Autodesk Fusion 360 part; units mm, degrees
sketch "Skizze1" plane through (0, 0, 0) normal (0, 0, 1) x (1, 0, 0)
  line L0 (-6.5, 4.75) -> (6.5, 4.75)
  line L1 (8.5, 2.75) -> (8.5, -2.75)
  line L2 (6.5, -4.75) -> (-6.5, -4.75)
  line L3 (-8.5, -2.75) -> (-8.5, 2.75)
  line L4 (-8.5, 4.75) -> (8.5, -4.75) construction
  line L5 (8.5, 4.75) -> (-8.5, -4.75) construction
  arc A0 (8.5, 2.75) -> (6.5, 4.75) centre (6.5, 2.75) ccw
  arc A1 (-6.5, 4.75) -> (-8.5, 2.75) centre (-6.5, 2.75) ccw
  arc A2 (-8.5, -2.75) -> (-6.5, -4.75) centre (-6.5, -2.75) ccw
  arc A3 (6.5, -4.75) -> (8.5, -2.75) centre (6.5, -2.75) ccw
  dimension "d464" = 17
  dimension "d465" = 9.5
  dimension "d468" = 2
extrude "Extrusion1" add sketch "Skizze1" along normal blind 2
sketch "Skizze2" plane through (0, 0, 2) normal (0, 0, 1) x (-1, 0, 0)
  arc A0 (8.5, 2.75) -> (6.5, 4.75) centre (6.5, 2.75) ccw
  line L0 (6.5, 4.75) -> (-6.5, 4.75)
  arc A1 (-6.5, 4.75) -> (-8.5, 2.75) centre (-6.5, 2.75) ccw
  line L1 (-8.5, 2.75) -> (-8.5, -2.75)
  arc A2 (-8.5, -2.75) -> (-6.5, -4.75) centre (-6.5, -2.75) ccw
  line L2 (-6.5, -4.75) -> (6.5, -4.75)
  arc A3 (6.5, -4.75) -> (8.5, -2.75) centre (6.5, -2.75) ccw
  line L3 (8.5, -2.75) -> (8.5, 2.75)
  line L4 (3.75, 2.25) -> (-3.75, 2.25)
  line L5 (-3.75, 2.25) -> (-3.75, -2.25)
  line L6 (-3.75, -2.25) -> (3.75, -2.25)
  line L7 (3.75, -2.25) -> (3.75, 2.25)
  line L8 (3.75, 2.25) -> (-3.75, -2.25) construction
  line L9 (-3.75, 2.25) -> (3.75, -2.25) construction
  dimension "d469" = 7.5
  dimension "d470" = 4.5
extrude "Extrusion2" add sketch "Skizze2" along normal blind 10 contours L4 L5 L6 L7
sketch "Skizze3" plane through (0, -2.25, 0) normal (0, -1, 0) x (1, 0, 0)
  line L0 (-3.75, 2) -> (3.75, 2)
  line L1 (3.75, 2) -> (3.75, 12)
  line L2 (3.75, 12) -> (-3.75, 12)
  line L3 (-3.75, 12) -> (-3.75, 2)
  line L4 (-0.875, 12) -> (0.875, 12)
  line L5 (0.875, 12) -> (0.875, 9)
  line L6 (0.875, 9) -> (-0.875, 9)
  line L7 (-0.875, 9) -> (-0.875, 12)
  line L8 (-0.875, 12) -> (0.875, 9) construction
  line L9 (0.875, 12) -> (-0.875, 9) construction
  line L10 (-3.75, 3.25) -> (-2.75, 4.25)
  line L11 (-3.75, 3.25) -> (-1.5, 3.25) construction
  line L12 (-2.75, 4.25) -> (-2.75, 5.75)
  line L13 (-2.75, 5.75) -> (-3.75, 6.75)
  line L14 (-6.5, 2) -> (6.5, 2)
  line L15 (0, 20) -> (0, 2.5)
  line L16 (3.75, 3.25) -> (2.75, 4.25)
  line L17 (2.75, 4.25) -> (2.75, 5.75)
  line L18 (2.75, 5.75) -> (3.75, 6.75)
  point P0 (0, 10.5)
  dimension "d479" = 1.75
  dimension "d480" = 3
  dimension "d483" = 45
  dimension "d484" = 1
  dimension "d485" = 1.5
  dimension "d486" = 2.25
extrude "Extrusion3" cut sketch "Skizze3" against normal up to surface (4.5 mm away) contours L3 L10 L12 L13 | L1 L16 L17 L18 | L2 L4 L6 L7 L15 | L2 L4 L5 L6 L15
sketch "Skizze4" plane through (0, 0, 0) normal (0, 0, -1) x (1, 0, 0)
  arc A0 (-6.5, 4.75) -> (-8.5, 2.75) centre (-6.5, 2.75) ccw
  line L0 (-8.5, 2.75) -> (-8.5, -2.75)
  arc A1 (-8.5, -2.75) -> (-6.5, -4.75) centre (-6.5, -2.75) ccw
  line L1 (-6.5, -4.75) -> (6.5, -4.75)
  arc A2 (6.5, -4.75) -> (8.5, -2.75) centre (6.5, -2.75) ccw
  line L2 (8.5, -2.75) -> (8.5, 2.75)
  arc A3 (8.5, 2.75) -> (6.5, 4.75) centre (6.5, 2.75) ccw
  line L3 (6.5, 4.75) -> (-6.5, 4.75)
  line L4 (-1, 3.5) -> (1, 3.5)
  line L5 (1, 3.5) -> (1, -3.5)
  line L6 (1, -3.5) -> (-1, -3.5)
  line L7 (-1, -3.5) -> (-1, 3.5)
  line L8 (-1, 3.5) -> (1, -3.5) construction
  line L9 (1, 3.5) -> (-1, -3.5) construction
  line L10 (-5.5, 3.5) -> (-3.5, 3.5)
  line L11 (-3.5, 3.5) -> (-3.5, -3.5)
  line L12 (-3.5, -3.5) -> (-5.5, -3.5)
  line L13 (-5.5, -3.5) -> (-5.5, 3.5)
  line L14 (-5.5, 3.5) -> (-3.5, -3.5) construction
  line L15 (-3.5, 3.5) -> (-5.5, -3.5) construction
  line L16 (3.5, 3.5) -> (5.5, 3.5)
  line L17 (5.5, 3.5) -> (5.5, -3.5)
  line L18 (5.5, -3.5) -> (3.5, -3.5)
  line L19 (3.5, -3.5) -> (3.5, 3.5)
  line L20 (3.5, 3.5) -> (5.5, -3.5) construction
  line L21 (5.5, 3.5) -> (3.5, -3.5) construction
  point P0 (-4.5, 0)
  point P1 (4.5, 0)
  dimension "d503" = 2
  dimension "d504" = 7
  dimension "d505" = 2.5
  dimension "d506" = 2.5
extrude "Extrusion4" cut sketch "Skizze4" against normal blind 0.5 contours L4 L5 L6 L7 | L10 L11 L12 L13 | L16 L17 L18 L19
chamfer "Fase1" distance 0.5 angle 45 12 edges at (-7.9142, -4.1642, 0) (0, -4.75, 0) (7.9142, -4.1642, 0) (8.5, 0, 0) (7.9142, 4.1642, 0) (0, 4.75, 0) (-7.9142, 4.1642, 0) (-8.5, 0, 0) (-2.3125, -2.25, 12) (2.3125, -2.25, 12) (-2.3125, 2.25, 12) (2.3125, 2.25, 12)
equation "d465 = 10 mm - ( 2 * 0.25 ) * 1 mm"
equation "d469 = 10 mm - 2.5 mm"
equation "d470 = 5 mm - ( 2 * 0.25 ) * 1 mm"
equation "d486 = 2 mm + 0.25 mm"
equation "d506 = d505"
The model under review builds one solid part; all positions refer to its coordinate system, in mm. A direction names the side the tool comes from. Coordinates: 2 decimals unless noted, no trailing zeros. Order: outer loops, then holes, each group sorted by start corner. A loop starts at its lowest first (then second) coordinate and runs counter-clockwise, first axis right, second up. Notation, with made-up numbers: (71.25, 15) -> (78.25, 15) arc R8 ccw to (78.25, 23) -> close; hole circle Ø6 at (82, -31.5). An arc over 180 degrees is marked (long way). Answer in a Markdown table with one row per item. Add a question column.
Item 1: Machinability: for faces 4 (the flat face through (3, 0, 4)), 5 (the flat face through (-5, 0, 0.5)), 6 (the flat face through (-3.75, 0, 3)), which of the approach directions +Z, -Z, +X, -X, +Y, -Y give a long, thin tool a straight path to every point of the face, cutting with its end or side? Answer none if there is none.
Item 2: We need section B-B on x = 5. Write out the cut boundary in (y, z), plus the area to 4 significant figures.
Item 3: Clearance check with flat-ended pins moving along their axes: pin 1 (1.6 mm diameter, centred on y = -0.5, z = 5, fed in from +X); pin 2 (0.6 mm diameter, centred on x = -5, z = 0, fed in from +Y); pin 3 (1.4 mm diameter, centred on y = -0.5, z = 3, fed in from +X). State where each tip first meets the part, or that it passes through.
Item 4: We need section A-A on z = 9.75. Write out the cut boundary in (x, y) (3 decimals), plus the area to 3 significant figures.
Item 5: Mouldability with a two-part tool opening along Z and no side actions: class faces 1 (the conical face through (7.67, 3.9, 0.14)), 2 (the flat face through (-2.75, 0, 5)), 3 (the flat face through (3.75, 0, 3)) as +Z half, -Z half, draft (parallel to the pull), parting line (faces both ways), or undercut.
Item 6: We need section D-D on z = 7.75. Write out the cut boundary in (x, y), plus the area to 4 significant figures.
Final values:
| question | item | result |
|---|---|---|
| 1 | face 4 | +X, +Y, -Y |
| 1 | face 5 | -Z |
| 1 | face 6 | +Z, -X, +Y, -Y |
| 2 | outline | (-4.75, 0.5) -> (-4.25, 0) -> (-3.5, 0) -> (-3.5, 0.5) -> (3.5, 0.5) -> (3.5, 0) -> (4.25, 0) -> (4.75, 0.5) -> (4.75, 2) -> (-4.75, 2) -> close |
| 2 | area | 15.25 mm2 |
| 3 | pin 1 | stops at x = 2.8 |
| 3 | pin 2 | stops at y = 4.55 |
| 3 | pin 3 | stops at x = 3.75 |
| 4 | outline | (-3.75, -2.25) -> (-0.875, -2.25) -> (-0.875, 2.25) -> (-3.75, 2.25) -> close; (0.875, -2.25) -> (3.75, -2.25) -> (3.75, 2.25) -> (0.875, 2.25) -> close |
| 4 | area | 25.9 mm2 |
| 5 | face 1 | -Z half |
| 5 | face 2 | undercut |
| 5 | face 3 | draft |
| 6 | outline | (-3.75, -2.25) -> (3.75, -2.25) -> (3.75, 2.25) -> (-3.75, 2.25) -> close |
| 6 | area | 33.75 mm2 |
